```python
from build123d import *

# Parameters (mm, degrees)
BOSS_EXTRUDE1_DEPTH = 50
CUT_EXTRUDE1_DEPTH  = 76
CUT_EXTRUDE2_DEPTH  = 59.548154505
BOSS_EXTRUDE2_REACH = 77
CUT_EXTRUDE3_DEPTH  = 100.601194791
SKETCH8_R           = 2.5
CUT_EXTRUDE4_DEPTH  = 100.601194791
SKETCH9_R           = 7.5
CUT_EXTRUDE5_DEPTH  = 40


with BuildPart() as part:
    # Sketch1 → Boss-Extrude1 (new body)
    with BuildSketch(Plane.XY):
        with BuildLine():
            Line((-15, 0), (-15, 5))
            Line((-15, 5), (-25, 5))
            Line((-25, 5), (-25, -25))
            Line((-25, -25), (25, -25))
            Line((25, -25), (25, 5))
            Line((25, 5), (15, 5))
            Line((15, 5), (15, -5))
            Line((15, -5), (19.364916731, -5))
            ThreePointArc((19.364916731, -5), (0, -20), (-19.364916731, -5))
            Line((-19.364916731, -5), (-15, -5))
            Line((-15, -5), (-15, 0))
        make_face()
    extrude(amount=BOSS_EXTRUDE1_DEPTH)

    # Sketch2 → Cut-Extrude1 (cut, through all)
    with BuildSketch(Plane(origin=(25, 0, 0), x_dir=(0, 0, -1), z_dir=(1, 0, 0))):
        Polygon((0, 5), (-7.155559798, 5), (0, -5.219198462), align=None)
        Polygon((-50, 5), (-50, -25), (-7.155559798, 5), align=None)
    extrude(amount=-CUT_EXTRUDE1_DEPTH, mode=Mode.SUBTRACT)

    # Sketch4 → Cut-Extrude2 (cut, through all)
    with BuildSketch(Plane(origin=(0, -1.717063728, 2.452221141), x_dir=(-1, 0, 0), z_dir=(0, 0.573576436351043, -0.8191520442889939))):
        Polygon((25, -4.27531709), (0, -29.27531709), (25, -29.27531709), align=None)
        Polygon((0, -29.27531709), (-25, -4.27531709), (-25, -29.27531709), align=None)
    extrude(amount=-CUT_EXTRUDE2_DEPTH, mode=Mode.SUBTRACT)

    # Boss-Extrude2: up to this face of the body (flat: up to its plane)
    boss_extrude2_end = Plane(part.part.faces().sort_by_distance((-25, -12.379979849, 21.845856759))[0])
    # Sketch6 → Boss-Extrude2 (add, up to the picked face)
    with BuildSketch(Plane(origin=(25, 0, 0), x_dir=(0, 0, -1), z_dir=(1, 0, 0)), mode=Mode.PRIVATE) as boss_extrude2_sk1:
        Polygon((-50, -25), (-74.574561329, -42.207293091), (-58.125064912, -65.69960861), (0, -25), align=None)
    boss_extrude2_tool1 = split(extrude(boss_extrude2_sk1.sketch, amount=-BOSS_EXTRUDE2_REACH, mode=Mode.PRIVATE), bisect_by=boss_extrude2_end, keep=Keep.BOTH, mode=Mode.PRIVATE)
    add(boss_extrude2_tool1.solids().sort_by(Axis((25, -40.270944, 43.428409), (-1, 0, 0)))[0])

    # Sketch7 → Cut-Extrude3 (cut, through all)
    with BuildSketch(Plane(origin=(0, -1.717063728, 2.452221141), x_dir=(-1, 0, 0), z_dir=(0, 0.573576436351043, -0.8191520442889939))):
        Polygon((25, -4.27531709), (25, -20.478801107), (8.796515983, -20.478801107), align=None)
        Polygon((-25, -4.27531709), (-8.796515983, -20.478801107), (-25, -20.478801107), align=None)
    extrude(amount=-CUT_EXTRUDE3_DEPTH, mode=Mode.SUBTRACT)

    # Sketch8 → Cut-Extrude4 (cut, through all)
    with BuildSketch(Plane(origin=(0, -1.717063728, 2.452221141), x_dir=(-1, 0, 0), z_dir=(0, 0.573576436351043, -0.8191520442889939))):
        with Locations(Location((0, -4.007725177, 0), (0, 0, 90))):
            Circle(SKETCH8_R)
    extrude(amount=-CUT_EXTRUDE4_DEPTH, mode=Mode.SUBTRACT)

    # Sketch9 → Cut-Extrude5 (cut)
    with BuildSketch(Plane(origin=(0, -1.717063728, 2.452221141), x_dir=(-1, 0, 0), z_dir=(0, 0.573576436351043, -0.8191520442889939))):
        with Locations(Location((0, -4.007725177, 0), (0, 0, 90))):
            Circle(SKETCH9_R)
    extrude(amount=-CUT_EXTRUDE5_DEPTH, mode=Mode.SUBTRACT)


solid = part.part
```
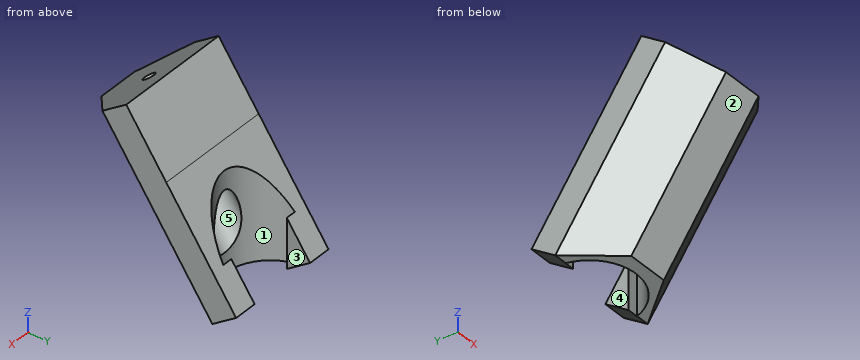
Geometry: final body of the model. Coordinates: model frame, mm. Face numbers are marked on the shaded views. A direction names the side the tool comes from. Round coordinates to 2 decimals unless told otherwise and drop trailing zeros. Order: outer loops, then holes, each group sorted by start corner. A loop starts at its lowest first (then second) coordinate and runs counter-clockwise, first axis right, second up. Notation, with made-up numbers: (-37, 13.5) -> (21, 13.5) arc R18 cw to (21, 22.5) -> close; hole circle Ø6 at (1.5, 16.25). An arc over 180 degrees is marked (long way). Use CSV: the item, a comma, the result in double quotes. Start each with the question number.
1) Section C-C (x = -21). Return the cut outline in (y, z), and give its area (3 significant figures).
2) Draft query along Y for the marked faces 1, 2 and 3. Return one class per face: +Y half, -Y half, draft (parallel to the pull), parting line (faces both ways), or undercut.
3) Material intervals for line 1 along X through (y, z) = (-44, 55.5); line 2 along X through (y, z) = (-44, 58); line 3 along Y through (x, z) = (2, 51), sorted ascending. Write a range as from..to.
4) Section B-B (x = -1.5). Return the cut outline in (y, z), and give its area (3 significant figures).
5) First-contact query: pin 1 Ø1.3 at (x, z) = (16.5, 15) entering from -Y; pin 2 Ø6 at (x, y) = (11.5, -29.5) entering from -Z; pin 3 Ø4 at (x, z) = (12, 27.5) entering from +Y. Flat tips, straight axial feed; report the tip coordinate or a pass-through.
6) Section D-D (y = -11.5). Return the cut outline in (x, z), and give its area (3 significant figures).
7) Section A-A (y = -1). Return the cut outline in (x, z), and give its area (3 significant figures).
8) Set-up query: the marked faces 4 and 5. Return all of +Z, -Z, +X, -X, +Y, -Y with unobstructed straight access to the full face (end or side cutting, diameter ignored); none if empty.
Returned:
1,outline,"(-55.7, 65.12) -> (-10.1, 0) -> (-5.22, 0) -> (5, 7.16) -> (-42.21, 74.57) -> close"
1,area,"1,350 mm²"
2,face 1,"undercut"
2,face 2,"-Y half"
2,face 3,"draft"
3,line 1,"x = -25..-2.49, 2.49..25"
3,line 2,"x = -25..-2.18, 2.18..25"
3,line 3,"y = -60.71..-42.43, -38.77..-25.7"
4,outline,"(-65.7, 58.13) -> (-25, 0) -> (-19.94, 0) -> (-19.94, 8.68) -> (-33.96, 28.7) -> (-29.58, 31.77) -> (-53.85, 66.43) -> close; (-50.57, 68.72) -> (-26.3, 34.07) -> (-21.92, 37.13) -> (-19.94, 34.31) -> (-19.94, 42.78) -> (-42.21, 74.57) -> close"
4,area,"1,310 mm²"
5,pin 1,"stops at y = -27.01"
5,pin 2,"stops at z = 4.38"
5,pin 3,"stops at y = -14.28"
6,outline,"(-25, 8.97) -> (-19.86, 0) -> (-16.36, 0) -> (-16.36, 30.72) -> (-25, 30.72) -> close; (16.36, 0) -> (19.86, 0) -> (25, 8.97) -> (25, 30.72) -> (16.36, 30.72) -> close"
6,area,"485 mm²"
7,outline,"(-25, 2.95) -> (-15, 2.95) -> (-15, 15.72) -> (-25, 15.72) -> close; (15, 2.95) -> (25, 2.95) -> (25, 15.72) -> (15, 15.72) -> close"
7,area,"255 mm²"
8,face 4,"+Z, -Z, +Y"
8,face 5,"none"
